from build123d import *


with BuildPart() as f1:
    # F0 (on Front) → F1 (revolve)
    with BuildSketch(Plane.XZ):
        with BuildLine():
            Line((-15.8, 8.07061), (-15.8, 0))
            Line((-15.8, 0), (-12.8, 0))
            Line((-12.8, 0), (-12.8, 8.07061))
            ThreePointArc((-12.8, 8.07061), (-12.674235, 8.374235), (-12.37061, 8.5))
            Line((-12.37061, 8.5), (0, 8.5))
            Line((0, 8.5), (0, 11.5))
            Line((0, 11.5), (-23, 11.5))
            Line((-23, 11.5), (-29, 11.5))
            Line((-29, 11.5), (-29, 8.5))
            Line((-29, 8.5), (-23, 8.5))
            Line((-23, 8.5), (-23, 0))
            Line((-23, 0), (-20, 0))
            Line((-20, 0), (-18.8, 1.134371))
            Line((-18.8, 1.134371), (-20, 1.134371))
            Line((-20, 1.134371), (-20, 8.07061))
            ThreePointArc((-20, 8.07061), (-19.874235, 8.374235), (-19.57061, 8.5))
            Line((-19.57061, 8.5), (-16.22939, 8.5))
            ThreePointArc((-16.22939, 8.5), (-15.925765, 8.374235), (-15.8, 8.07061))
        make_face()
    revolve(axis=Axis((0, 0, 10), (0, 0, -1)))


solid = f1.part
Here's how the part is built. I have some questions about the finished solid (model axes, mm). A direction names the side the tool comes from. Coordinates: 2 decimals unless noted, no trailing zeros. Loops run counter-clockwise (first coordinate to the right, second up) from the corner with the lowest first, then second, coordinate; pieces in that order, holes last.
1. For P1, Ø1.5, axis at x = 16.5, z = 9, coming from the +Y side; P2, Ø12.5, axis at x = 0.5, y = -1.5, coming from the -Z side; P3, Ø4, axis at y = 4.5, z = 3, coming from the +X side, each with a flat end and sliding along its axis, tell me the tip position at first contact or that it passes through.
2. Imagine slicing it at B-B, the plane z = 6.25. Please give me the cut outline in (x, y), and give its area (3 significant figures).
3. For faces 5 (the cylindrical face through (12.54, -9.61, 3.98)), 6 (the flat face through (-13, 0, 0)), 7 (the flat face through (7, 15, 8.5)), which set-ups out of +Z, -Z, +X, -X, +Y, -Y let a thin tool reach every point of the face, with its end or its side?
4. I need wall thicknesses on L1, parallel to Y at x = 0, z = 3; L2, parallel to Y at x = -1, z = 0.75; L3, parallel to X at y = -13, z = 3.25. Which ranges of each line are inside material? Lowest first, please.
5. If we mould it in two halves opening along Z, with no side actions, what happens to faces 1 (the flat face through (0, 0, 8.5)), 2 (the flat face through (15, -12, 1.134)), 3 (the cylindrical face through (4.336, -19.524, 4.651)), 4 (the cylindrical face through (-13.38, -25.73, 9.98))? For each: pulls with the +Z half, pulls with the -Z half, needs draft (parallel to the pull), parting line crosses it, or undercut.
Taken from the geometry:
1. P1: stops at y = 24.35
1. P2: stops at z = 8.5
1. P3: stops at x = 22.86
2. outline: circle Ø46 at (0, 0); circle Ø31.6 at (0, 0); hole circle Ø40 at (0, 0); hole circle Ø25.6 at (0, 0)
2. area: 675 mm2
3. face 5: -Z
3. face 6: -Z, +X, -X, +Y, -Y
3. face 7: none
4. L1: y = -23 to -20, -15.8 to -12.8, 12.8 to 15.8, 20 to 23
4. L2: y = -22.98 to -19.18, -15.77 to -12.76, 12.76 to 15.77, 19.18 to 22.98
4. L3: x = -18.97 to -15.2, -8.98 to 8.98, 15.2 to 18.97
5. face 1: pulls with the -Z half
5. face 2: undercut
5. face 3: undercut
5. face 4: needs draft
